```python
from build123d import *

# Parameters (mm, degrees)
F0_W     = 180
F0_H     = 60
F1_DEPTH = 25
F2_W     = 25
F2_H     = 60
F3_DEPTH = 87
F4_R     = 29.99999
F5_SIZE  = 15
F6_R     = 18
F7_DEPTH = 25
F8_R     = 10
F9_DEPTH = 25.001


# Not quite as in the source:
# - a fillet or chamfer is up to 0.001 mm smaller than in the source, because OpenCascade refuses the exact size


with BuildPart() as f1:
    # F0 (on Top) → F1 (new body)
    with BuildSketch(Plane.XY):
        with Locations((90, 30)):
            Rectangle(F0_W, F0_H)
    extrude(amount=F1_DEPTH)

    # F2 (on face) → F3 (join)
    with BuildSketch(Plane.XY.offset(25)):
        with Locations((12.5, 30)):
            Rectangle(F2_W, F2_H)
    extrude(amount=F3_DEPTH)

    # F4 (radius 30 in the source; OpenCascade refuses exactly that, so slightly less here)
    f4_edges = [f1.edges().sort_by_distance(p)[0] for p in [
        (12.5, 0, 112),
        (12.5, 60, 112),
    ]]
    fillet(f4_edges, radius=F4_R)

    # F5
    f5_edges = [f1.edges().sort_by_distance(p)[0] for p in [
        (180, 0, 12.5),
        (180, 60, 12.5),
    ]]
    chamfer(f5_edges, length=F5_SIZE)

    # F6 (on face) → F7 (cut)
    with BuildSketch(Plane.XY.offset(25)):
        with Locations((70, 30)):
            Circle(F6_R)
        with Locations((135, 30)):
            Circle(F6_R)
    extrude(amount=-F7_DEPTH, mode=Mode.SUBTRACT)

    # F8 (on face) → F9 (cut, through all)
    with BuildSketch(Plane.YZ.offset(25)):
        with Locations((30, 82)):
            Circle(F8_R)
    extrude(amount=-F9_DEPTH, mode=Mode.SUBTRACT)


solid = f1.part
```
CAD build for the part. Positions are in the model's coordinates, mm. A direction names the side the tool comes from. Round coordinates to 2 decimals unless told otherwise and drop trailing zeros. Loops run counter-clockwise (first coordinate to the right, second up) from the corner with the lowest first, then second, coordinate; pieces in that order, holes last. Notation, with made-up numbers: M 87,51.25 L 141,51.25 A29 ccw 141,82.25 Z; hole C 50,88 d4. An arc over 180 degrees is marked long. Use a Markdown table: item, result. Add a question column.
(1) Flat gauge pins, fed straight in: pin 1 (8 mm diameter, centred on y = 41.5, z = 80, fed in from +X); pin 2 (4 mm diameter, centred on x = 27.5, y = 42.5, fed in from +Z); pin 3 (18 mm diameter, centred on y = 30, z = 82, fed in from -X). Where does each tip first touch, or does it go through?
(2) Pull direction Y, two halves, no side cores. Call faces 3 (the face through (63, 60, 22)), 4 (the face through (173, 8, 12)), 5 (the face through (12.68, 35.38, 90.43)): +Y half, -Y half, draft (parallel to the pull), parting line (faces both ways), or undercut.
(3) Cut at C-C (z = 37). Give the cut face in (x, y), and give its area (3 significant figures).
(4) Which spindle directions (+Z, -Z, +X, -X, +Y, -Y) get a long thin tool onto all of the face, cutting with end or side? Do faces 1 (the face through (52.017, 30.791, 12.675)), 2 (the face through (25, 30, 68)). Say none if no direction does.
(5) Cut at A-A (x = 70). Give the cut face in (y, z), and give its area (3 significant figures).
(6) Drill centre lines: line 1 (Y direction, x = 70, z = 18); line 2 (Z direction, x = 17, y = 30); line 3 (X direction, y = 46.5, z = 65.5). Where is each one in solid material? Low to high.
(7) Cut at D-D (x = 128.5). Give the cut face in (y, z).
(8) Cut at B-B (y = 23). Give the cut face in (x, z), and give its area (3 significant figures).
Geometry says:
| question | item | result |
|---|---|---|
| 1 | pin 1 | stops at x = 25 |
| 1 | pin 2 | stops at z = 25 |
| 1 | pin 3 | passes through |
| 2 | face 3 | +Y half |
| 2 | face 4 | -Y half |
| 2 | face 5 | undercut |
| 3 | outline | M 0,0 L 25,0 L 25,60 L 0,60 Z |
| 3 | area | 1,500 mm² |
| 4 | face 1 | +Z, -Z |
| 4 | face 2 | +Z, +X, +Y, -Y |
| 5 | outline | M 0,0 L 12,0 L 12,25 L 0,25 Z; M 48,0 L 60,0 L 60,25 L 48,25 Z |
| 5 | area | 600 mm² |
| 6 | line 1 | y = 0 to 12, 48 to 60 |
| 6 | line 2 | z = 0 to 72, 92 to 112 |
| 6 | line 3 | x = 0 to 25 |
| 7 | outline | M 0,0 L 13.21,0 L 13.21,25 L 0,25 Z; M 46.79,0 L 60,0 L 60,25 L 46.79,25 Z |
| 8 | outline | M 0,0 L 53.42,0 L 53.42,25 L 25,25 L 25,74.86 L 0,74.86 Z; M 0,89.14 L 25,89.14 L 25,111.17 L 0,111.17 Z; M 86.58,0 L 118.42,0 L 118.42,25 L 86.58,25 Z; M 151.58,0 L 180,0 L 180,25 L 151.58,25 Z |
| 8 | area | 4,640 mm² |
